from build123d import *

# Parameters (mm, degrees)
F0_R     = 2.54
F1_DEPTH = 76.2
F3_DEPTH = 1.27
F4_DEPTH = 1.27


with BuildPart() as f1:
    # F0 (on Top) → F1 (new body)
    with BuildSketch(Plane.XY):
        Circle(F0_R)
    extrude(amount=F1_DEPTH)

    # F2 (on Front) → F3 (join)
    with BuildSketch(Plane.XZ):
        Polygon((19.7582356632, 69.153830409), (0, 69.153830409), (0, 46.79011181), (11.0732968897, 46.79011181), (11.0732968897, 48.5270991921), (13.6787788942, 48.5270991921), (13.6787788942, 46.79011181), (20.19248344, 46.79011181), (20.19248344, 50.2640865743), (6.7308279686, 50.2640865743), (6.7308279686, 54.6065531671), (21.2781019509, 54.6065531671), (21.2781019509, 59.1661445796), (16.5013838559, 59.1661445796), (16.5013838559, 57.212036103), (11.0732968897, 57.212036103), (11.0732968897, 59.1661445796), (6.7308279686, 59.1661445796), (6.7308279686, 65.0284811854), (19.7582356632, 65.0284811854), align=None)
    extrude(amount=F3_DEPTH)

    # F2 (on Front) → F4 (join)
    with BuildSketch(Plane.XZ):
        Polygon((19.7582356632, 69.153830409), (0, 69.153830409), (0, 46.79011181), (11.0732968897, 46.79011181), (11.0732968897, 48.5270991921), (13.6787788942, 48.5270991921), (13.6787788942, 46.79011181), (20.19248344, 46.79011181), (20.19248344, 50.2640865743), (6.7308279686, 50.2640865743), (6.7308279686, 54.6065531671), (21.2781019509, 54.6065531671), (21.2781019509, 59.1661445796), (16.5013838559, 59.1661445796), (16.5013838559, 57.212036103), (11.0732968897, 57.212036103), (11.0732968897, 59.1661445796), (6.7308279686, 59.1661445796), (6.7308279686, 65.0284811854), (19.7582356632, 65.0284811854), align=None)
    extrude(amount=-F4_DEPTH)


solid = f1.part
Input: part model. Units: mm. Frame: model coordinates. A direction names the side the tool comes from. Coordinates: 2 decimals unless noted, no trailing zeros. Loops run counter-clockwise (first coordinate to the right, second up) from the corner with the lowest first, then second, coordinate; pieces in that order, holes last. Notation, with made-up numbers: (61.25, 87.5) -> (70.25, 87.5) arc R15 cw to (70.25, 98.5) -> close; hole circle Ø5 at (-16.75, -31). An arc over 180 degrees is marked (long way). Write each question's results on one line, items separated by ' | '. Start each with the question number.
Q1. Section C-C, the plane z = 49.5. Return the cut outline in (x, y), plus the area to 3 significant figures.
Q2. Pin query (flat end, axial travel): pin 1 (2 mm diameter, centred on x = 14.5, y = 0.5, fed in from +Z); pin 2 (2 mm diameter, centred on y = -0.5, z = 49, fed in from +X); pin 3 (2 mm diameter, centred on y = 0.5, z = 67.5, fed in from +X). Return the tip coordinate at first contact, or that it passes through.
Q3. Reachability of faces 4 (the flat face through (20.192, 0, 49)), 5 (the flat face through (14, 0, 57.212)), 6 (the flat face through (13, 0, 65.028)) from +Z, -Z, +X, -X, +Y, -Y: full face, straight path, thin tool, end or side. Return the list, or none.
Q4. Ray query, line 1 (Z direction, x = 12, y = -1.1); line 2 (Z direction, x = 7, y = -1.05); line 3 (Z direction, x = 20.25, y = -0.5). Return the intervals inside material, ascending. Write a range as from..to.
Q5. Section D-D, the plane x = 6. Return the cut outline in (y, z).
Q6. Pull-direction query (Z, two-part tool) for faces 1 (the cylindrical face through (-2.538, 0.112, 37.567)), 2 (the flat face through (17, 0, 46.79)), 3 (the flat face through (6.731, 0, 52)); classes: released by +Z, released by -Z, zero draft, split by the parting line, or undercut.
Q7. Section B-B, the plane y = 0. Return the cut outline in (x, z), plus the area to 3 significant figures.
Q8. Section A-A, the plane x = 9.5. Return the cut outline in (y, z).
Found:
1) outline: (2.2, -1.27) -> (20.19, -1.27) -> (20.19, 1.27) -> (2.2, 1.27) arc R2.54 ccw (long way) to start | area: 65.4 mm2
2) pin 1: z = 69.15 | pin 2: x = 20.19 | pin 3: x = 19.76
3) face 4: -Z, +X, +Y, -Y | face 5: +Y, -Y | face 6: +X, +Y, -Y
4) line 1: 48.53..50.26, 54.61..57.21, 65.03..69.15 | line 2: 46.79..50.26, 54.61..59.17, 65.03..69.15 | line 3: 54.61..59.17
5) outline: (-1.27, 46.79) -> (1.27, 46.79) -> (1.27, 69.15) -> (-1.27, 69.15) -> close
6) face 1: zero draft | face 2: released by -Z | face 3: undercut
7) outline: (-2.54, 0) -> (2.54, 0) -> (2.54, 46.79) -> (11.07, 46.79) -> (11.07, 48.53) -> (13.68, 48.53) -> (13.68, 46.79) -> (20.19, 46.79) -> (20.19, 50.26) -> (6.73, 50.26) -> (6.73, 54.61) -> (21.28, 54.61) -> (21.28, 59.17) -> (16.5, 59.17) -> (16.5, 57.21) -> (11.07, 57.21) -> (11.07, 59.17) -> (6.73, 59.17) -> (6.73, 65.03) -> (19.76, 65.03) -> (19.76, 69.15) -> (2.54, 69.15) -> (2.54, 76.2) -> (-2.54, 76.2) -> close | area: 633 mm2
8) outline: (-1.27, 46.79) -> (1.27, 46.79) -> (1.27, 50.26) -> (-1.27, 50.26) -> close; (-1.27, 54.61) -> (1.27, 54.61) -> (1.27, 59.17) -> (-1.27, 59.17) -> close; (-1.27, 65.03) -> (1.27, 65.03) -> (1.27, 69.15) -> (-1.27, 69.15) -> close
